Can you work these out from the model? Positions are in its coordinate system, mm. A direction names the side the tool comes from. Coordinates: 2 decimals unless noted, no trailing zeros. Order: outer loops, then holes, each group sorted by start corner. A loop starts at its lowest first (then second) coordinate and runs counter-clockwise, first axis right, second up. Notation, with made-up numbers: (-32, -39) -> (-20, -39) arc R20 ccw to (-20, -6) -> close; hole circle Ø5 at (89, -38). An arc over 180 degrees is marked (long way). Answer in a Markdown table with one row per item. Add a question column.
1. Imagine slicing it at C-C on y = 76.2. State how many separate pieces and enclosed holes the cut face has, plus the area to 3 significant figures.
2. Imagine slicing it at A-A on x = -33. Write out the boundary of the cut face in (y, z).
3. Imagine slicing it at B-B on y = 13. Write out the boundary of the cut face in (x, z).
4. On a 3-axis mill with a long thin cutter (end or side, diameter ignored), from which of +Z, -Z, +X, -X, +Y, -Y can I reach the whole of each face in a straight line? I mean faces 1 (the face through (-102, 56, 27.05)), 2 (the face through (-101.6, -4, 24)), 3 (the face through (-31, 125, 9)), 4 (the face through (-124.4, 43, 13)), 5 (the face through (-114.3, -4, 24)). Say none if no direction works.
5. We'd pull the mould along X, two halves only. Please class faces 6 (the face through (-76.935, 42.704, 17.527)), 7 (the face through (-152.4, 35, 18)), 8 (the face through (-104.819, 78.346, 24.71)): pulls with the +X half, pulls with the -X half, needs draft (parallel to the pull), parting line crosses it, or undercut.
6. Will these pins go through, and if not, where does the flat tip stop? pin 1 (12 mm diameter, centred on x = -88.5, z = 21.5, fed in from +Y); pin 2 (18.5 mm diameter, centred on x = -44, z = 17, fed in from -Y); pin 3 (5 mm diameter, centred on x = -88, z = 23.5, fed in from -Y); pin 4 (6 mm diameter, centred on x = -34, y = 51, fed in from -Z).
7. If I drill on line 1 along X through (y, z) = (105, 21.5); line 2 along Y through (x, z) = (-106, 27); line 3 along X through (y, z) = (56, 26.5), over which ranges is the centre line in solid material (lowest first)? Write a range as [from, to].
from build123d import *

# Parameters (mm, degrees)
SALIENTE_EXTRUIR1_DEPTH = 54.1
REDONDEO1_R             = 10
CROQUIS2_W              = 27.05
CROQUIS2_H              = 127
CORTAR_EXTRUIR1_DEPTH   = 206.624828267
VACIADO1_T              = -4
CROQUIS3_W              = 22.730580246
CROQUIS3_H              = 69.392963169
SALIENTE_EXTRUIR2_DEPTH = 5
CROQUIS3_3_W            = 5
CROQUIS3_3_H            = 50
CROQUIS3_3_H_2          = 35
SALIENTE_EXTRUIR3_DEPTH = 18
CROQUIS4_W              = 5
CROQUIS4_H              = 32.000123075
SALIENTE_EXTRUIR4_DEPTH = 23.05
CORTAR_EXTRUIR2_REACH   = 185.317
CROQUIS5_R              = 9.525
CROQUIS6_W              = 38.1
CROQUIS6_H              = 42.277753805
CORTAR_EXTRUIR3_DEPTH   = 18
CROQUIS7_W              = 180.240941947
CROQUIS7_H              = 148.875136133
CORTAR_EXTRUIR4_DEPTH   = 201.216039567
SALIENTE_EXTRUIR5_DEPTH = 12.7
CROQUIS9_R              = 1.5875
CORTAR_EXTRUIR5_DEPTH   = 174.832338789
CROQUIS10_R             = 3.175
SALIENTE_EXTRUIR6_DEPTH = 6.35


with BuildPart() as part:
    # Croquis1 → Saliente-Extruir1 (new body)
    with BuildSketch(Plane.XY):
        Polygon((0, 0), (0, 127), (63.5, 127), (63.5, 69.85), (152.4, 69.85), (152.4, 0), align=None)
    extrude(amount=SALIENTE_EXTRUIR1_DEPTH)

    # Redondeo1
    redondeo1_edges = [part.edges().sort_by_distance(p)[0] for p in [
        (63.5, 69.85, 27.05),
        (152.4, 69.85, 27.05),
        (152.4, 0, 27.05),
        (0, 0, 27.05),
        (152.4, 34.925, 0),
    ]]
    fillet(redondeo1_edges, radius=REDONDEO1_R)

    # Croquis2 → Cortar-Extruir1 (cut, through all)
    with BuildSketch(Plane(origin=(152.4, 0, 0), x_dir=(0, 0, -1), z_dir=(1, 0, 0))):
        with Locations((-40.575, 63.5)):
            Rectangle(CROQUIS2_W, CROQUIS2_H)
    extrude(amount=-CORTAR_EXTRUIR1_DEPTH, mode=Mode.SUBTRACT)

    # Vaciado1
    vaciado1_openings = [part.faces().sort_by_distance(p)[0] for p in [
        (64.737748774, 51.223088278, 27.05),
    ]]
    offset(amount=VACIADO1_T, openings=vaciado1_openings)

    # Croquis3 → Saliente-Extruir2 (add)
    with BuildSketch(Plane.XY.offset(4)):
        with Locations((31.75, 72.216754897)):
            Rectangle(CROQUIS3_W, CROQUIS3_H)
    extrude(amount=SALIENTE_EXTRUIR2_DEPTH)

    # Croquis3<3> → Saliente-Extruir3 (add)
    with BuildSketch(Plane.XY.offset(4)):
        with Locations((10.184709877, 77.438130808)):
            Rectangle(CROQUIS3_3_W, CROQUIS3_3_H)
        with Locations((53.315290123, 88.988130808)):
            Rectangle(CROQUIS3_3_W, CROQUIS3_3_H_2)
        Polygon((50.815290123, 20.688130808), (43.115290123, 20.688130808), (43.115290123, 15.688130808), (55.815290123, 15.688130808), (55.815290123, 28.388130808), (50.815290123, 28.388130808), align=None)
        Polygon((20.384709877, 20.688130808), (12.684709877, 20.688130808), (12.684709877, 28.388130808), (7.684709877, 28.388130808), (7.684709877, 15.688130808), (20.384709877, 15.688130808), align=None)
    extrude(amount=SALIENTE_EXTRUIR3_DEPTH)

    # Croquis4 → Saliente-Extruir4 (add)
    with BuildSketch(Plane.XY.offset(4)):
        with Locations((76.9, 42.913130808)):
            Rectangle(CROQUIS4_W, CROQUIS4_H)
        with Locations((101.9, 42.913130808)):
            Rectangle(CROQUIS4_W, CROQUIS4_H)
        with Locations((126.9, 42.913130808)):
            Rectangle(CROQUIS4_W, CROQUIS4_H)
    extrude(amount=SALIENTE_EXTRUIR4_DEPTH)

    # Cortar-Extruir2: up to this face of the body (flat: up to its plane)
    cortar_extruir2_end = Plane(part.part.faces().sort_by_distance((55.815290123, 22.038130808, 13))[0])
    # Croquis5 → Cortar-Extruir2 (cut, up to the picked face)
    with BuildSketch(Plane(origin=(129.4, 0, 0), x_dir=(0, 0, -1), z_dir=(1, 0, 0)), mode=Mode.PRIVATE) as cortar_extruir2_sk1:
        with Locations((-27.05, 42.913130808)):
            Circle(CROQUIS5_R)
    cortar_extruir2_tool1 = split(extrude(cortar_extruir2_sk1.sketch, amount=-CORTAR_EXTRUIR2_REACH, mode=Mode.PRIVATE), bisect_by=cortar_extruir2_end, keep=Keep.BOTH, mode=Mode.PRIVATE)
    add(cortar_extruir2_tool1.solids().sort_by(Axis((129.4, 42.913131, 27.05), (-1, 0, 0)))[0], mode=Mode.SUBTRACT)

    # Croquis6 → Cortar-Extruir3 (cut)
    with BuildSketch(Plane.XZ.offset(-123)):
        with Locations((31.75, 30.138876903)):
            Rectangle(CROQUIS6_W, CROQUIS6_H)
    extrude(amount=-CORTAR_EXTRUIR3_DEPTH, mode=Mode.SUBTRACT)

    # Simetría5: part across plane


with BuildPart() as part_1:
    add(part.part)
    add(part.part.mirror(Plane(origin=(0, 0, 54.1), x_dir=(0, 0, 1), z_dir=(1, 0, 0))))

    # Croquis7 → Cortar-Extruir4 (cut, through all)
    with BuildSketch(Plane.XY.offset(27.05)):
        with Locations((90.120470974, 52.562431934)):
            Rectangle(CROQUIS7_W, CROQUIS7_H)
    extrude(amount=-CORTAR_EXTRUIR4_DEPTH, mode=Mode.SUBTRACT)

    # Croquis8 → Saliente-Extruir5 (add)
    with BuildSketch(Plane(origin=(-38.1, 0, 0), x_dir=(0, 0, -1), z_dir=(1, 0, 0))):
        with BuildLine():
            Line((-27.05, 0), (-17.144, 0))
            Line((-17.144, 0), (-23.0876, -7.9248))
            ThreePointArc((-23.0876, -7.9248), (-31.480097877, -7.168048939), (-27.05, 0))
        make_face()
    saliente_extruir5 = extrude(amount=-SALIENTE_EXTRUIR5_DEPTH)

    # Croquis9 → Cortar-Extruir5 (cut, through all)
    with BuildSketch(Plane(origin=(-38.1, 0, 0), x_dir=(0, 0, -1), z_dir=(1, 0, 0))):
        with Locations((-27.05, -4.953)):
            Circle(CROQUIS9_R)
    cortar_extruir5 = extrude(amount=-CORTAR_EXTRUIR5_DEPTH, mode=Mode.SUBTRACT)

    # Simetría6: Saliente-Extruir5, Cortar-Extruir5 across plane
    add(saliente_extruir5.mirror(Plane(origin=(-76.2, 0, 0), x_dir=(0, 0, 1), z_dir=(1, 0, 0))))
    add(cortar_extruir5.mirror(Plane(origin=(-76.2, 0, 0), x_dir=(0, 0, 1), z_dir=(1, 0, 0))), mode=Mode.SUBTRACT)

    # Croquis10 → Saliente-Extruir6 (add)
    with BuildSketch(Plane.ZY.offset(107.95)):
        with BuildLine():
            Line((27.05, 69.85), (14.35, 69.85))
            Line((14.35, 69.85), (21.97, 80.01))
            ThreePointArc((21.97, 80.01), (32.729612663, 79.039806331), (27.05, 69.85))
        make_face()
        with Locations((27.05, 76.2)):
            Circle(CROQUIS10_R, mode=Mode.SUBTRACT)
    extrude(amount=-SALIENTE_EXTRUIR6_DEPTH)


solid = part_1.part
Answers follow:
| question | item | result |
|---|---|---|
| 1 | separate pieces | 3 |
| 1 | enclosed holes | 0 |
| 1 | area | 790 mm² |
| 2 | outline | (0, 0) -> (127, 0) -> (127, 9) -> (123, 9) -> (123, 4) -> (106.91, 4) -> (106.91, 9) -> (37.52, 9) -> (37.52, 4) -> (4, 4) -> (4, 27.05) -> (0, 27.05) -> close |
| 3 | outline | (-152.4, 10) arc R10 ccw to (-142.4, 0) -> (0, 0) -> (0, 27.05) -> (-4, 27.05) -> (-4, 4) -> (-142.4, 4) arc R6 cw to (-148.4, 10) -> (-148.4, 27.05) -> (-152.4, 27.05) -> close |
| 4 | face 1 | +Z, +X, -X |
| 4 | face 2 | +Z, -Z, -Y |
| 4 | face 3 | +Z, +Y |
| 4 | face 4 | +Z |
| 4 | face 5 | +Z, -Z, -X, -Y |
| 5 | face 6 | undercut |
| 5 | face 7 | pulls with the -X half |
| 5 | face 8 | needs draft |
| 6 | pin 1 | stops at y = 69.85 |
| 6 | pin 2 | stops at y = -9.84 |
| 6 | pin 3 | stops at y = 0 |
| 6 | pin 4 | stops at z = 0 |
| 7 | line 1 | x = [-63.5, -59.5], [-55.82, -50.82], [-4, 0] |
| 7 | line 2 | y = [-9.91, -6.54], [-3.37, 4], [65.85, 73.03], [79.37, 82.55] |
| 7 | line 3 | x = [-152.4, -148.4], [-129.4, -124.4], [-104.4, -99.4], [-79.4, -74.4], [-4, 0] |
